```python
from build123d import *

# Parameters (mm, degrees)
SKETCH_1_W               = 11
SKETCH_1_H               = 10.9642
CUT_EXTRUDE_2_REACH      = 24.345
PATTERN_CIRCULAR_3_COUNT = 18
SKETCH_7_R               = 30
EXTRUDE_1_DEPTH          = 6
SKETCH_8_R               = 2.7888
EXTRUDE_2_DEPTH          = 11
SKETCH_10_R              = 11
CUT_EXTRUDE_3_DEPTH      = 2
SKETCH_11_R              = 1.6
CUT_EXTRUDE_4_DEPTH      = 44.829214002
PATTERN_CIRCULAR_4_COUNT = 3
SKETCH_13_R              = 1.975
CUT_EXTRUDE_5_DEPTH      = 44.829214002
CHAMFER_1_SIZE           = 0.8
CHAMFER_2_SIZE           = 2.5
CUT_EXTRUDE_START        = -15
SKETCH_14_R              = 4
CUT_EXTRUDE_6_DEPTH      = 10
SKETCH_15_R              = 4.5
CUT_EXTRUDE_7_DEPTH      = 46.705579528
CHAMFER_3_SIZE           = 2
SKETCH_17_R              = 6.025
CUT_EXTRUDE_8_DEPTH      = 3.5
CUT_EXTRUDE_START_2      = -3.4
SKETCH_18_R              = 6.025
CUT_EXTRUDE_9_DEPTH      = 3.4


with BuildPart() as part:
    # 草图1 → 旋转1 (revolve)
    with BuildSketch(Plane.XY, mode=Mode.PRIVATE) as revolve_1_sk:
        with Locations((5.5, 8.2709)):
            Rectangle(SKETCH_1_W, SKETCH_1_H)
    revolve(revolve_1_sk.sketch.rotate(Axis((0, 0, 0), (1, 0, 0)), 90), axis=Axis((0, 0, 0), (1, 0, 0)))

    # 草图6 → 切除-拉伸2 (cut, up to next)
    with BuildSketch(Plane(origin=(0, 0, 0), x_dir=(0, 0, -1), z_dir=(1, 0, 0)), mode=Mode.PRIVATE) as cut_extrude_2_sk1:
        with BuildLine():
            Line((1.574067282, 13.17215513), (1.548371997, 12.962883824))
            ThreePointArc((1.548371997, 12.962883824), (0, 11.593), (-1.548371997, 12.962883824))
            Line((-1.548371997, 12.962883824), (-1.574067282, 13.17215513))
            ThreePointArc((-1.574067282, 13.17215513), (-1.761240253, 13.496717776), (-2.124642597, 13.587895453))
            ThreePointArc((-2.124642597, 13.587895453), (-2.36143787, 13.548749765), (-2.597513963, 13.505477785))
            Line((-2.597513963, 13.505477785), (-2.794161951, 15.107047128))
            ThreePointArc((-2.794161951, 15.107047128), (0, 15.363274844), (2.794161951, 15.107047128))
            Line((2.794161951, 15.107047128), (2.597513963, 13.505477785))
            ThreePointArc((2.597513963, 13.505477785), (2.36143787, 13.548749765), (2.124642597, 13.587895453))
            ThreePointArc((2.124642597, 13.587895453), (1.761240253, 13.496717776), (1.574067282, 13.17215513))
        make_face()
    cut_extrude_2_tool1 = extrude(cut_extrude_2_sk1.sketch, amount=CUT_EXTRUDE_2_REACH, mode=Mode.PRIVATE) & part.part
    cut_extrude_2 = cut_extrude_2_tool1.solids().sort_by_distance((0, 13.819423, 0))[0]
    add(cut_extrude_2, mode=Mode.SUBTRACT)

    # 阵列(圆周)3: 切除-拉伸2 ×18 about axis
    pattern_circular_3_axis = Axis((0, 0, 0), (1, 0, 0))
    for i in range(1, PATTERN_CIRCULAR_3_COUNT):
        add(cut_extrude_2.rotate(pattern_circular_3_axis, i * 360 / PATTERN_CIRCULAR_3_COUNT), mode=Mode.SUBTRACT)

    # 草图7 → 凸台-拉伸1 (add)
    with BuildSketch(Plane(origin=(11, 0, 0), x_dir=(0, 0, -1), z_dir=(1, 0, 0))):
        Circle(SKETCH_7_R)
    extrude(amount=EXTRUDE_1_DEPTH)

    # 草图8 → 凸台-拉伸2 (add)
    with BuildSketch(Plane.ZY):
        Circle(SKETCH_8_R)
    extrude(amount=-EXTRUDE_2_DEPTH)

    # 草图10 → 切除-拉伸3 (cut)
    with BuildSketch(Plane(origin=(17, 0, 0), x_dir=(0, 0, -1), z_dir=(1, 0, 0))):
        Circle(SKETCH_10_R)
    extrude(amount=-CUT_EXTRUDE_3_DEPTH, mode=Mode.SUBTRACT)

    # 草图11 → 切除-拉伸4 (cut, through all)
    with BuildSketch(Plane.ZY.offset(-11)):
        with Locations((0, 20)):
            Circle(SKETCH_11_R)
    cut_extrude_4 = extrude(amount=-CUT_EXTRUDE_4_DEPTH, mode=Mode.SUBTRACT)

    # 阵列(圆周)4: 切除-拉伸4 ×3 about axis
    pattern_circular_4_axis = Axis((0, 0, 0), (1, 0, 0))
    for i in range(1, PATTERN_CIRCULAR_4_COUNT):
        add(cut_extrude_4.rotate(pattern_circular_4_axis, i * 360 / PATTERN_CIRCULAR_4_COUNT), mode=Mode.SUBTRACT)

    # 草图13 → 切除-拉伸5 (cut, through all)
    with BuildSketch(Plane.ZY.offset(-11)):
        with Locations((17.320508076, 10)):
            Circle(SKETCH_13_R)
    extrude(amount=-CUT_EXTRUDE_5_DEPTH, mode=Mode.SUBTRACT)

    # 倒角1
    chamfer_1_edges = [part.edges().sort_by_distance(p)[0] for p in [
        (11, 10, 15.345508076),
    ]]
    chamfer(chamfer_1_edges, length=CHAMFER_1_SIZE)

    # 倒角2
    chamfer_2_edges = [part.edges().sort_by_distance(p)[0] for p in [
        (11, 20, -1.6),
        (11, -8.614359354, 18.120508076),
        (11, -11.385640646, -16.520508076),
    ]]
    chamfer(chamfer_2_edges, length=CHAMFER_2_SIZE)

    # 草图14 → 切除-拉伸6 (cut)
    with BuildSketch(Plane.ZY.offset(CUT_EXTRUDE_START)):
        with Locations(Location((0, 0, 0), (0, 0, 180))):
            Circle(SKETCH_14_R)
    extrude(amount=CUT_EXTRUDE_6_DEPTH, mode=Mode.SUBTRACT)

    # 草图15 → 切除-拉伸7 (cut, through all)
    with BuildSketch(Plane.ZY):
        Circle(SKETCH_15_R)
    extrude(amount=-CUT_EXTRUDE_7_DEPTH, mode=Mode.SUBTRACT)

    # 倒角3
    chamfer_3_edges = [part.edges().sort_by_distance(p)[0] for p in [
        (11, 0, 30),
    ]]
    chamfer(chamfer_3_edges, length=CHAMFER_3_SIZE)

    # 草图17 → 切除-拉伸8 (cut)
    with BuildSketch(Plane(origin=(15, 0, 0), x_dir=(0, 0, -1), z_dir=(1, 0, 0))):
        Circle(SKETCH_17_R)
    extrude(amount=-CUT_EXTRUDE_8_DEPTH, mode=Mode.SUBTRACT)

    # 草图18 → 切除-拉伸9 (cut)
    with BuildSketch(Plane.ZY.offset(CUT_EXTRUDE_START_2)):
        with Locations(Location((0, 0, 0), (0, 0, 180))):
            Circle(SKETCH_18_R)
    extrude(amount=CUT_EXTRUDE_9_DEPTH, mode=Mode.SUBTRACT)


solid = part.part
```
Read the model definition and answer for the solid it produces. Units are mm, in the model's axes. A direction names the side the tool comes from. Give positions to 0.01 mm unless a question says otherwise; leave off trailing zeros. One line per item, written item: value. Start each with the question number.
(1) The part is cut by section A-A (z = 0). State how many separate pieces and enclosed holes the cut face has, and give its area (3 significant figures).
(2) Flat-ended cylindrical pins translate along their axes: P1, Ø1.9, axis at y = 20, z = 0, coming from the +X side; P2, Ø9.5, axis at y = 2.5, z = -0.5, coming from the +X side; P3, Ø1, axis at x = 12, y = -19, coming from the +Z side; P4, Ø5, axis at x = 2, y = 1.5, coming from the -Z side. Find the tip coordinate at first contact, or state that the pin passes through.
(3) Straight lines are drawn through the part: L1, parallel to Y at x = 13.6, z = 0 (3 decimals); L2, parallel to Y at x = 8, z = 0; L3, parallel to X at y = -22, z = -6. For each, find the intervals that lie inside material, in ascending order.
(4) A tool of negligible diameter and unlimited length cuts with its end or side. For faces 1 (the cylindrical face through (15.226, 21.586, -0.208)), 2 (the cylindrical face through (1.72, -4.07, 4.44)), 3 (the cylindrical face through (13.27, 4.07, 4.44)), 4 (the cylindrical face through (5.423, 11.593, -0.032)), from which of +Z, -Z, +X, -X, +Y, -Y can it reach the whole face along a straight path? Write none if from no direction.
Taken from the geometry:
1. separate pieces: 3
1. enclosed holes: 0
1. area: 386 mm^2
2. P1: through
2. P2: x = 15
2. P3: z = 22.69
2. P4: z = -13.75
3. L1: -30 to -6.025, 6.025 to 18.4, 21.6 to 30
3. L2: -11.59 to -4.5, 4.5 to 11.59
3. L3: 11 to 17
4. face 1: +X, -X
4. face 2: -X
4. face 3: +X
4. face 4: -X, +Y
